Model file for the job. Use its own axes, mm. Coordinates: 2 decimals unless noted, no trailing zeros. Order: outer loops, then holes, each group sorted by start corner. A loop starts at its lowest first (then second) coordinate and runs counter-clockwise, first axis right, second up.
from build123d import *

# Parameters (mm, degrees)
EXTRUDE_1_DEPTH = 2


with BuildPart() as part:
    # 草图1 → 凸台-拉伸1 (new body)
    with BuildSketch(Plane(origin=(0, 0, 0), x_dir=(1, 0, 0), z_dir=(0, 1, 0))):
        with BuildLine():
            Line((12.924395537, 2.4), (15.570240846, 2.4))
            ThreePointArc((15.570240846, 2.4), (17.165195809, 3.193302579), (17.494868886, 4.943881335))
            ThreePointArc((17.494868886, 4.943881335), (13.110639725, 12.594583201), (5.642066631, 17.282346025))
            ThreePointArc((5.642066631, 17.282346025), (4.744501657, 17.141149105), (4.331721931, 16.331721931))
            ThreePointArc((4.331721931, 16.331721931), (0, 12), (-4.331721931, 16.331721931))
            ThreePointArc((-4.331721931, 16.331721931), (-4.744501657, 17.141149105), (-5.642066631, 17.282346025))
            ThreePointArc((-5.642066631, 17.282346025), (-13.110639725, 12.594583201), (-17.494868886, 4.943881335))
            ThreePointArc((-17.494868886, 4.943881335), (-17.165195809, 3.193302579), (-15.570240846, 2.4))
            Line((-15.570240846, 2.4), (-12.924395537, 2.4))
            ThreePointArc((-12.924395537, 2.4), (-12.18018713, 2.067947488), (-11.930211265, 1.292307692))
            ThreePointArc((-11.930211265, 1.292307692), (-11.850930243, -1.885590724), (-10.94, -4.931166191))
            Line((-10.94, -4.931166191), (-15.165520228, -12.249981915))
            ThreePointArc((-15.165520228, -12.249981915), (-16.833795519, -13.248964827), (-18.56235636, -12.358354517))
            ThreePointArc((-18.56235636, -12.358354517), (0, 22.3), (18.56235636, -12.358354517))
            ThreePointArc((18.56235636, -12.358354517), (16.833795519, -13.248964827), (15.165520228, -12.249981915))
            Line((15.165520228, -12.249981915), (10.94, -4.931166191))
            ThreePointArc((10.94, -4.931166191), (11.850930243, -1.885590724), (11.930211265, 1.292307692))
            ThreePointArc((11.930211265, 1.292307692), (12.18018713, 2.067947488), (12.924395537, 2.4))
        make_face()
    extrude(amount=EXTRUDE_1_DEPTH)


solid = part.part
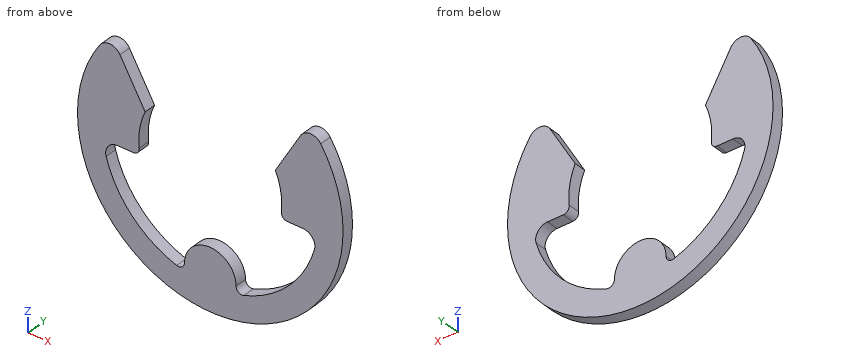
Q1. Probe line 1 (Z direction, x = -16, y = 1.95); line 2 (X direction, y = 0.4, z = 6); line 3 (Z direction, x = 14.5, y = 0.6). List the from-to ranges inside material, lowest first.
Established:
line 1: z = -15.53 to -8.63, -2.45 to 13.04
line 2: x = -21.48 to -11.56, 11.56 to 21.48
line 3: z = -16.94 to -10.97, -2.4 to 11.1
Q2. Cut at C-C, the plane y = 0.9. List the corners of the cut face in (x, z), plus the area to 3 significant figures.
Established:
outline: (-18.56, 12.36) arc R22.3 ccw (long way) to (18.56, 12.36) arc R2 ccw to (15.17, 12.25) - (10.94, 4.93) arc R12 cw to (11.93, -1.29) arc R1 ccw to (12.92, -2.4) - (15.57, -2.4) arc R2 cw to (17.49, -4.94) arc R18.18 cw to (5.64, -17.28) arc R1 cw to (4.33, -16.33) arc R4.33 ccw to (-4.33, -16.33) arc R1 cw to (-5.64, -17.28) arc R18.18 cw to (-17.49, -4.94) arc R2 cw to (-15.57, -2.4) - (-12.92, -2.4) arc R1 ccw to (-11.93, -1.29) arc R12 cw to (-10.94, 4.93) - (-15.17, 12.25) arc R2 ccw to start
area: 555 mm2
Q3. Drop flat-ended pins along their axis: P1, Ø5, axis at x = 14.5, z = 4.5, coming from the -Y side; P2, Ø1, axis at y = 1, z = 4, coming from the -X side; P3, Ø1, axis at x = 15, y = 1.5, coming from the -Z side. Give the stop position or say it passes through.
Established:
P1: stops at y = 0
P2: stops at x = -22.02
P3: stops at z = -16.94
Q4. Cut at A-A, the plane z = 9. List the corners of the cut face in (x, y).
Established:
outline: (-20.4, 0) - (-13.29, 0) - (-13.29, 2) - (-20.4, 2) - close; (13.29, 0) - (20.4, 0) - (20.4, 2) - (13.29, 2) - close
Q5. Cut at D-D, the plane z = 3.5. List the corners of the cut face in (x, y).
Established:
outline: (-22.02, 0) - (-11.48, 0) - (-11.48, 2) - (-22.02, 2) - close; (11.48, 0) - (22.02, 0) - (22.02, 2) - (11.48, 2) - close
Q6. Cut at B-B, the plane z = -12.5. List the corners of the cut face in (x, y), plus the area to 3 significant figures.
Established:
outline: (-18.47, 0) - (-13.2, 0) - (-13.2, 2) - (-18.47, 2) - close; (-2.02, 0) - (2.02, 0) - (2.02, 2) - (-2.02, 2) - close; (13.2, 0) - (18.47, 0) - (18.47, 2) - (13.2, 2) - close
area: 29.1 mm2
